Answer from the drawing. Dimensions are ordinates in mm from the lowest x, y and z of the part. A direction names the side the tool comes from. Give positions to 0.01 mm unless a question says otherwise; leave off trailing zeros. Write each loop counter-clockwise with the first axis right and the second up, starting at its lowest first coordinate (ties: lowest second). Pieces come first, ordered by that corner, then holes. Notation, with made-up numbers: M 52.25,-14.75 L 102.25,-14.75 A17 ccw 102.25,4.25 Z; hole C -9,14.5 d7. An arc over 180 degrees is marked long. Put each result on its own line as item: value.
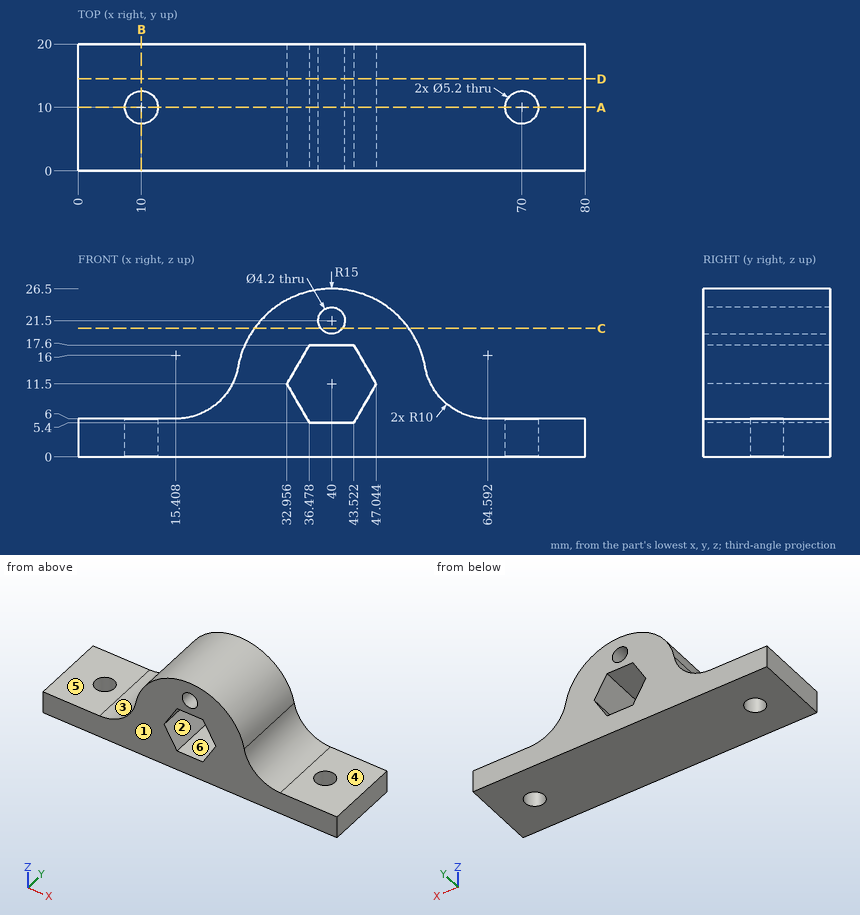
(1) Section C-C on z = 20.25 is taken. Determine the outline of the cut face in (x, y).
Result:
outline: M 27.82,0 L 38.31,0 L 38.31,20 L 27.82,20 Z; M 41.69,0 L 52.18,0 L 52.18,20 L 41.69,20 Z
(2) Which of the six approach directions +Z, -Z, +X, -X, +Y, -Y give full straight-line access (tool end or side, diameter ignored) to the marked faces 4, 5 and 6?
Result:
face 4: +Z, +X, +Y, -Y
face 5: +Z, -X, +Y, -Y
face 6: +Y, -Y
(3) Straight lines are drawn through the part: line 1 along Z through (x, y) = (4.5, 6.25); line 2 along Y through (x, z) = (70, 3.15); line 3 along X through (y, z) = (4, 21.5). For each, find the intervals that lie inside material, in ascending order. Write a range as from..to.
Result:
line 1: z = 0..6
line 2: y = 0..7.4, 12.6..20
line 3: x = 28.82..37.9, 42.1..51.18
(4) For a pull along X with two mould halves and no side action, classify the marked faces 1, 2 and 3 as +X half, -X half, draft (parallel to the pull), parting line (faces both ways), or undercut.
Result:
face 1: draft
face 2: undercut
face 3: -X half
(5) Section A-A on y = 10 is taken. Determine the outline of the cut face in (x, z) (1 decimal).
Result:
outline: M 0,0 L 7.4,0 L 7.4,6 L 0,6 Z; M 12.6,0 L 67.4,0 L 67.4,6 L 64.6,6 A10 cw 54.8,14.2 A15 ccw 25.2,14.2 A10 cw 15.4,6 L 12.6,6 Z; M 72.6,0 L 80,0 L 80,6 L 72.6,6 Z; hole M 33,11.5 L 36.5,5.4 L 43.5,5.4 L 47,11.5 L 43.5,17.6 L 36.5,17.6 Z; hole C 40,21.5 d4.2
(6) Given pin 1 Ø1 at (y, z) = (15, 13.5) entering from -X; pin 2 Ø7.5 at (x, y) = (10, 13) entering from +Z; pin 3 Ø10 at (y, z) = (8, 18.5) entering from +X; pin 4 Ø3.5 at (x, z) = (40, 21.5) entering from +Y, each flat-ended and moving along its own axis, determine where each tip first touches the part or whether it passes through.
Result:
pin 1: stops at x = 24.95
pin 2: stops at z = 6
pin 3: stops at x = 54.91
pin 4: passes through
(7) Section B-B on x = 10 is taken. Determine the outline of the cut face in (y, z), and give its area (3 significant figures).
Result:
outline: M 0,0 L 7.4,0 L 7.4,6 L 0,6 Z; M 12.6,0 L 20,0 L 20,6 L 12.6,6 Z
area: 88.8 mm²
(8) Section D-D on y = 14.5 is taken. Determine the outline of the cut face in (x, z) (1 decimal), and give its area (3 significant figures).
Result:
outline: M 0,0 L 80,0 L 80,6 L 64.6,6 A10 cw 54.8,14.2 A15 ccw 25.2,14.2 A10 cw 15.4,6 L 0,6 Z; hole M 33,11.5 L 36.5,5.4 L 43.5,5.4 L 47,11.5 L 43.5,17.6 L 36.5,17.6 Z; hole C 40,21.5 d4.2
area: 892 mm²
